from build123d import *

# Parameters (mm, degrees)
F1_DEPTH = 150


with BuildPart() as f1:
    # F0 (on Right) → F1 (new body)
    with BuildSketch(Plane.YZ):
        with BuildLine():
            Line((-43.745468, 0.644926), (-21.125, -10))
            Line((-21.125, -10), (-21.125, 15))
            ThreePointArc((-21.125, 15), (-34.520463, 11.108329), (-43.745468, 0.644926))
        make_face()
        Polygon((-16.125, -10), (-16.125, 10), (16.125, 10), (16.125, -10), (21.125, -10), (21.125, 15), (-21.125, 15), (-21.125, -10), align=None)
    extrude(amount=F1_DEPTH)

    # F2 (on face) → F3 (revolve, cut)
    with BuildSketch(Plane(origin=(0, -7.68272, -16.325779), x_dir=(1, 0, 0), z_dir=(0, -0.425797, -0.904819))):
        with BuildLine():
            Line((54, 22.356325), (46, 22.356325))
            ThreePointArc((46, 22.356325), (43.5, 19.856325), (46, 17.356325))
            Line((46, 17.356325), (54, 17.356325))
            ThreePointArc((54, 17.356325), (56.5, 19.856325), (54, 22.356325))
        make_face()
        with BuildLine():
            Line((104, 22.356325), (96, 22.356325))
            ThreePointArc((96, 22.356325), (93.5, 19.856325), (96, 17.356325))
            Line((96, 17.356325), (104, 17.356325))
            ThreePointArc((104, 17.356325), (106.5, 19.856325), (104, 22.356325))
        make_face()
    revolve(axis=Axis((75, -32.435234, -4.677537), (1, 0, 0)), mode=Mode.SUBTRACT)


solid = f1.part
Work out the finished part from the listing and answer in its coordinate system (mm). A direction names the side the tool comes from. Give positions to 0.01 mm unless a question says otherwise; leave off trailing zeros. Loops run counter-clockwise (first coordinate to the right, second up) from the corner with the lowest first, then second, coordinate; pieces in that order, holes last. Notation, with made-up numbers: M 25,-35.75 L 30,-35.75 A14 ccw 30,-19.75 Z; hole C 16.25,-20 d6. An arc over 180 degrees is marked long. Use CSV: the item, a comma, the result in double quotes.
1) Find section C-C on y = 6. Write down the section's boundary in (x, z), plus the area to 3 significant figures.
Answer:
outline,"M 0,10 L 150,10 L 150,15 L 0,15 Z"
area,"750 mm^2"
2) Determine the mould class of faces 1 (the flat face through (0, -19, 5)), 2 (the cylindrical face through (100.056, -27.979, 4.275)), 3 (the cylindrical face through (49.94, -30.21, -0.2)), 4 (the flat face through (74, 0, 15)) for opening direction X: released by +X, released by -X, zero draft, split by the parting line, or undercut.
Answer:
face 1,"released by -X"
face 2,"undercut"
face 3,"undercut"
face 4,"zero draft"
3) Consider L1, parallel to Y at x = 53, z = -1.5 (1 decimal); L2, parallel to Z at x = 77.5, y = 10.5; L3, parallel to Y at x = 76.5, z = -6.75 (3 decimals). Determine where each line is inside the solid, lowest interval first.
Answer:
L1,"-36.3 to -28.6, -23 to -16.1, 16.1 to 21.1"
L2,"10 to 15"
L3,"-28.031 to -16.125, 16.125 to 21.125"
4) Find section A-A on z = 7. Write down the section's boundary in (x, y) (3 decimals), plus the area to 3 significant figures.
Answer:
outline,"M 0,-39.455 L 150,-39.455 L 150,-16.125 L 0,-16.125 Z; M 0,16.125 L 150,16.125 L 150,21.125 L 0,21.125 Z"
area,"4,250 mm^2"
5) Find section D-D on y = -35.5. Give the number of separate pieces and of enclosed holes in the cut face, plus the area to 3 significant figures.
Answer:
separate pieces,"1"
enclosed holes,"2"
area,"1,920 mm^2"
6) Which of the six approach directions +Z, -Z, +X, -X, +Y, -Y give full straight-line access (tool end or side, diameter ignored) to faces 5 (the flat face through (74, -19, -10)), 6 (the cylindrical face through (50.056, -27.979, 4.275)), 7 (the flat face through (74, 16.125, 0))?
Answer:
face 5,"-Z, +X, -X, +Y, -Y"
face 6,"none"
face 7,"-Z, +X, -X"
7) Given P1, Ø16, axis at x = 84.5, y = 5, coming from the -Z side; P2, Ø6, axis at x = 130, y = -30.5, coming from the -Z side; P3, Ø1.5, axis at x = 48, y = -26, coming from the -Z side, each flat-ended and moving along its own axis, determine where each tip first touches the part or whether it passes through.
Answer:
P1,"z = 10"
P2,"z = -7"
P3,"z = 2.28"
8) Find section B-B on x = 21.5. Write down the section's boundary in (y, z) (3 decimals).
Answer:
outline,"M -43.745,0.645 L -21.125,-10 L -16.125,-10 L -16.125,10 L 16.125,10 L 16.125,-10 L 21.125,-10 L 21.125,15 L -21.125,15 A25 ccw Z"
